from build123d import *

# Parameters (mm, degrees)
BOX014_W     = 100
BOX014_H     = 10
BOX014_DEPTH = 120
FILLET_R     = 50
FILLET001_R  = 50


with BuildPart() as part:
    # Box014 → Box014 (new body)
    with BuildSketch(Plane(origin=(-10, -46, 0), x_dir=(1, 0, 0), z_dir=(0, 0, 1))):
        with Locations((50, 5)):
            Rectangle(BOX014_W, BOX014_H)
    extrude(amount=BOX014_DEPTH)

    # Fillet
    fillet_edges = [part.edges().sort_by_distance(p)[0] for p in [
        (90, -41, 0),
    ]]
    fillet(fillet_edges, radius=FILLET_R)

    # Fillet001
    fillet001_edges = [part.edges().sort_by_distance(p)[0] for p in [
        (90, -41, 120),
    ]]
    fillet(fillet001_edges, radius=FILLET001_R)


solid = part.part
Here's how the part is built. I have some questions about the finished solid (model axes, mm). Round coordinates to 2 decimals unless told otherwise and drop trailing zeros. Loops run counter-clockwise (first coordinate to the right, second up) from the corner with the lowest first, then second, coordinate; pieces in that order, holes last. Notation, with made-up numbers: (85, -36.75) - (100, -36.75) arc R8 ccw to (100, -25.75) - close; hole circle Ø6 at (35, 79). An arc over 180 degrees is marked (long way). One line per question, with ' | ' between items. Start each with the question number.
Q1. I want a section at C-C (x = 56.5). Write out the boundary of the cut face in (y, z).
Q2. Will these pins go through, and if not, where does the flat tip stop? pin 1 (2 mm diameter, centred on x = 58.5, y = -42, fed in from +Z); pin 2 (2 mm diameter, centred on x = 68, y = -40, fed in from -Z); pin 3 (5 mm diameter, centred on x = 42, y = -44.5, fed in from -Z); pin 4 (2 mm diameter, centred on x = 67.5, y = -37, fed in from -Z).
Q3. I want a section at A-A (y = -38.5). Write out the boundary of the cut face in (x, z).
Q4. I want a section at B-B (z = 22.5). Write out the boundary of the cut face in (x, y), then the cut area to 3 significant figures.
Q5. Please list where these lines run through material, in increasing order: line 1 (X direction, y = -38.25, z = 25.5); line 2 (X direction, y = -44, z = 81.5); line 3 (Z direction, x = 56.5, y = -38.75). Write a range as [from, to].
Response values:
1) outline: (-46, 2.8) - (-36, 2.8) - (-36, 117.2) - (-46, 117.2) - close
2) pin 1: stops at z = 116.84 | pin 2: stops at z = 7.92 | pin 3: stops at z = 0 | pin 4: stops at z = 7.6
3) outline: (-10, 0) - (40, 0) arc R50 ccw to (90, 50) - (90, 70) arc R50 ccw to (40, 120) - (-10, 120) - close
4) outline: (-10, -46) - (81.76, -46) - (81.76, -36) - (-10, -36) - close | area: 918 mm²
5) line 1: x = [-10, 83.59] | line 2: x = [-10, 88.66] | line 3: z = [2.8, 117.2]
